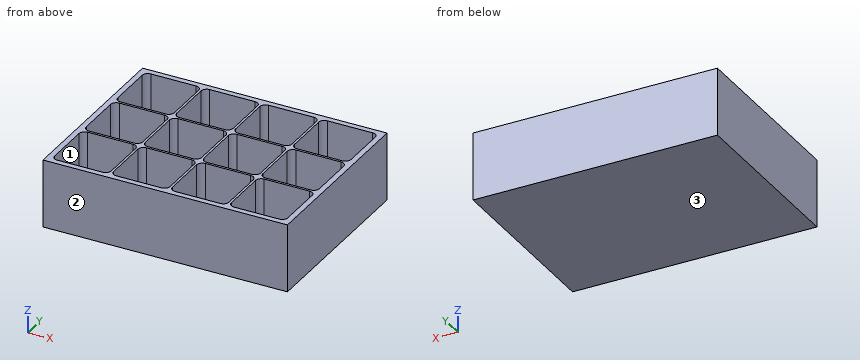
from build123d import *

# Parameters (mm, degrees)
F0_W     = 216
F0_H     = 164
F1_DEPTH = 60
F3_DEPTH = 58


with BuildPart() as f1:
    # F0 (on Top) → F1 (new body)
    with BuildSketch(Plane.XY):
        with Locations((3.771866, 32.061749)):
            Rectangle(F0_W, F0_H)
    extrude(amount=F1_DEPTH)

    # F2 (on face) → F3 (cut)
    with BuildSketch(Plane.XY.offset(60)):
        with BuildLine():
            ThreePointArc((-99.228134, -39.938251), (-97.763668, -43.473785), (-94.228134, -44.938251))
            Line((-94.228134, -44.938251), (-54.228134, -44.938251))
            ThreePointArc((-54.228134, -44.938251), (-50.6926, -43.473785), (-49.228134, -39.938251))
            Line((-49.228134, -39.938251), (-49.228134, 0.061749))
            ThreePointArc((-49.228134, 0.061749), (-50.6926, 3.597283), (-54.228134, 5.061749))
            Line((-54.228134, 5.061749), (-94.228134, 5.061749))
            ThreePointArc((-94.228134, 5.061749), (-97.763668, 3.597283), (-99.228134, 0.061749))
            Line((-99.228134, 0.061749), (-99.228134, -39.938251))
        make_face()
        with BuildLine():
            ThreePointArc((-54.228134, 7.061749), (-50.6926, 8.526215), (-49.228134, 12.061749))
            Line((-49.228134, 12.061749), (-49.228134, 52.061749))
            ThreePointArc((-49.228134, 52.061749), (-50.6926, 55.597283), (-54.228134, 57.061749))
            Line((-54.228134, 57.061749), (-94.228134, 57.061749))
            ThreePointArc((-94.228134, 57.061749), (-97.763668, 55.597283), (-99.228134, 52.061749))
            Line((-99.228134, 52.061749), (-99.228134, 12.061749))
            ThreePointArc((-99.228134, 12.061749), (-97.763668, 8.526215), (-94.228134, 7.061749))
            Line((-94.228134, 7.061749), (-54.228134, 7.061749))
        make_face()
        with BuildLine():
            ThreePointArc((-54.228134, 59.061749), (-50.6926, 60.526215), (-49.228134, 64.061749))
            Line((-49.228134, 64.061749), (-49.228134, 104.061749))
            ThreePointArc((-49.228134, 104.061749), (-50.6926, 107.597283), (-54.228134, 109.061749))
            Line((-54.228134, 109.061749), (-94.228134, 109.061749))
            ThreePointArc((-94.228134, 109.061749), (-97.763668, 107.597283), (-99.228134, 104.061749))
            Line((-99.228134, 104.061749), (-99.228134, 64.061749))
            ThreePointArc((-99.228134, 64.061749), (-97.763668, 60.526215), (-94.228134, 59.061749))
            Line((-94.228134, 59.061749), (-54.228134, 59.061749))
        make_face()
        with BuildLine():
            ThreePointArc((-2.228134, -44.938251), (1.3074, -43.473785), (2.771866, -39.938251))
            Line((2.771866, -39.938251), (2.771866, 0.061749))
            ThreePointArc((2.771866, 0.061749), (1.3074, 3.597283), (-2.228134, 5.061749))
            Line((-2.228134, 5.061749), (-42.228134, 5.061749))
            ThreePointArc((-42.228134, 5.061749), (-45.763668, 3.597283), (-47.228134, 0.061749))
            Line((-47.228134, 0.061749), (-47.228134, -39.938251))
            ThreePointArc((-47.228134, -39.938251), (-45.763668, -43.473785), (-42.228134, -44.938251))
            Line((-42.228134, -44.938251), (-2.228134, -44.938251))
        make_face()
        with BuildLine():
            ThreePointArc((-2.228134, 7.061749), (1.3074, 8.526215), (2.771866, 12.061749))
            Line((2.771866, 12.061749), (2.771866, 52.061749))
            ThreePointArc((2.771866, 52.061749), (1.3074, 55.597283), (-2.228134, 57.061749))
            Line((-2.228134, 57.061749), (-42.228134, 57.061749))
            ThreePointArc((-42.228134, 57.061749), (-45.763668, 55.597283), (-47.228134, 52.061749))
            Line((-47.228134, 52.061749), (-47.228134, 12.061749))
            ThreePointArc((-47.228134, 12.061749), (-45.763668, 8.526215), (-42.228134, 7.061749))
            Line((-42.228134, 7.061749), (-2.228134, 7.061749))
        make_face()
        with BuildLine():
            ThreePointArc((-2.228134, 59.061749), (1.3074, 60.526215), (2.771866, 64.061749))
            Line((2.771866, 64.061749), (2.771866, 104.061749))
            ThreePointArc((2.771866, 104.061749), (1.3074, 107.597283), (-2.228134, 109.061749))
            Line((-2.228134, 109.061749), (-42.228134, 109.061749))
            ThreePointArc((-42.228134, 109.061749), (-45.763668, 107.597283), (-47.228134, 104.061749))
            Line((-47.228134, 104.061749), (-47.228134, 64.061749))
            ThreePointArc((-47.228134, 64.061749), (-45.763668, 60.526215), (-42.228134, 59.061749))
            Line((-42.228134, 59.061749), (-2.228134, 59.061749))
        make_face()
        with BuildLine():
            ThreePointArc((49.771866, -44.938251), (53.3074, -43.473785), (54.771866, -39.938251))
            Line((54.771866, -39.938251), (54.771866, 0.061749))
            ThreePointArc((54.771866, 0.061749), (53.3074, 3.597283), (49.771866, 5.061749))
            Line((49.771866, 5.061749), (9.771866, 5.061749))
            ThreePointArc((9.771866, 5.061749), (6.236332, 3.597283), (4.771866, 0.061749))
            Line((4.771866, 0.061749), (4.771866, -39.938251))
            ThreePointArc((4.771866, -39.938251), (6.236332, -43.473785), (9.771866, -44.938251))
            Line((9.771866, -44.938251), (49.771866, -44.938251))
        make_face()
        with BuildLine():
            ThreePointArc((49.771866, 7.061749), (53.3074, 8.526215), (54.771866, 12.061749))
            Line((54.771866, 12.061749), (54.771866, 52.061749))
            ThreePointArc((54.771866, 52.061749), (53.3074, 55.597283), (49.771866, 57.061749))
            Line((49.771866, 57.061749), (9.771866, 57.061749))
            ThreePointArc((9.771866, 57.061749), (6.236332, 55.597283), (4.771866, 52.061749))
            Line((4.771866, 52.061749), (4.771866, 12.061749))
            ThreePointArc((4.771866, 12.061749), (6.236332, 8.526215), (9.771866, 7.061749))
            Line((9.771866, 7.061749), (49.771866, 7.061749))
        make_face()
        with BuildLine():
            ThreePointArc((49.771866, 59.061749), (53.3074, 60.526215), (54.771866, 64.061749))
            Line((54.771866, 64.061749), (54.771866, 104.061749))
            ThreePointArc((54.771866, 104.061749), (53.3074, 107.597283), (49.771866, 109.061749))
            Line((49.771866, 109.061749), (9.771866, 109.061749))
            ThreePointArc((9.771866, 109.061749), (6.236332, 107.597283), (4.771866, 104.061749))
            Line((4.771866, 104.061749), (4.771866, 64.061749))
            ThreePointArc((4.771866, 64.061749), (6.236332, 60.526215), (9.771866, 59.061749))
            Line((9.771866, 59.061749), (49.771866, 59.061749))
        make_face()
        with BuildLine():
            ThreePointArc((101.771866, -44.938251), (105.3074, -43.473785), (106.771866, -39.938251))
            Line((106.771866, -39.938251), (106.771866, 0.061749))
            ThreePointArc((106.771866, 0.061749), (105.3074, 3.597283), (101.771866, 5.061749))
            Line((101.771866, 5.061749), (61.771866, 5.061749))
            ThreePointArc((61.771866, 5.061749), (58.236332, 3.597283), (56.771866, 0.061749))
            Line((56.771866, 0.061749), (56.771866, -39.938251))
            ThreePointArc((56.771866, -39.938251), (58.236332, -43.473785), (61.771866, -44.938251))
            Line((61.771866, -44.938251), (101.771866, -44.938251))
        make_face()
        with BuildLine():
            ThreePointArc((101.771866, 7.061749), (105.3074, 8.526215), (106.771866, 12.061749))
            Line((106.771866, 12.061749), (106.771866, 52.061749))
            ThreePointArc((106.771866, 52.061749), (105.3074, 55.597283), (101.771866, 57.061749))
            Line((101.771866, 57.061749), (61.771866, 57.061749))
            ThreePointArc((61.771866, 57.061749), (58.236332, 55.597283), (56.771866, 52.061749))
            Line((56.771866, 52.061749), (56.771866, 12.061749))
            ThreePointArc((56.771866, 12.061749), (58.236332, 8.526215), (61.771866, 7.061749))
            Line((61.771866, 7.061749), (101.771866, 7.061749))
        make_face()
        with BuildLine():
            ThreePointArc((101.771866, 59.061749), (105.3074, 60.526215), (106.771866, 64.061749))
            Line((106.771866, 64.061749), (106.771866, 104.061749))
            ThreePointArc((106.771866, 104.061749), (105.3074, 107.597283), (101.771866, 109.061749))
            Line((101.771866, 109.061749), (61.771866, 109.061749))
            ThreePointArc((61.771866, 109.061749), (58.236332, 107.597283), (56.771866, 104.061749))
            Line((56.771866, 104.061749), (56.771866, 64.061749))
            ThreePointArc((56.771866, 64.061749), (58.236332, 60.526215), (61.771866, 59.061749))
            Line((61.771866, 59.061749), (101.771866, 59.061749))
        make_face()
    extrude(amount=-F3_DEPTH, mode=Mode.SUBTRACT)


solid = f1.part
The listing builds one solid part. Answer for the finished solid, in the listing's coordinates (mm). Face numbers are marked on the shaded views. Coordinates: 2 decimals unless noted, no trailing zeros. Loops run counter-clockwise (first coordinate to the right, second up) from the corner with the lowest first, then second, coordinate; pieces in that order, holes last.
1) Find section C-C on z = 7. Give the number of separate pieces and of enclosed holes in the cut face, then the cut area to 3 significant figures.
2) Find the intervals of material crossed by L1, parallel to Y at x = 91, z = 3.5; L2, parallel to X at y = 14.5, z = 24; L3, parallel to Y at x = 102.5, z = 43, in increasing order.
3) Find section A-A on y = 14.5. Write down the section's boundary in (x, z).
4) A flat-ended cylindrical pin translates along its axis: pin 1 Ø5 at (x, y) = (-12.5, 63) entering from +Z. Find the tip coordinate at first contact, or state that the pin passes through.
5) Determine the mould class of the marked faces 1, 2 and 3 for opening direction Y: pulls with the +Y half, pulls with the -Y half, needs draft (parallel to the pull), parting line crosses it, or undercut.
6) Find section B-B on x = -34.5. Write down the section's boundary in (y, z).
Values:
1. separate pieces: 1
1. enclosed holes: 12
1. area: 5,680 mm2
2. L1: y = -49.94 to -44.94, 5.06 to 7.06, 57.06 to 59.06, 109.06 to 114.06
2. L2: x = -104.23 to -99.23, -49.23 to -47.23, 2.77 to 4.77, 54.77 to 56.77, 106.77 to 111.77
2. L3: y = -49.94 to -44.88, 5.01 to 7.12, 57.01 to 59.12, 109.01 to 114.06
3. outline: (-104.23, 0) - (111.77, 0) - (111.77, 60) - (106.77, 60) - (106.77, 2) - (56.77, 2) - (56.77, 60) - (54.77, 60) - (54.77, 2) - (4.77, 2) - (4.77, 60) - (2.77, 60) - (2.77, 2) - (-47.23, 2) - (-47.23, 60) - (-49.23, 60) - (-49.23, 2) - (-99.23, 2) - (-99.23, 60) - (-104.23, 60) - close
4. pin 1: stops at z = 2
5. face 1: undercut
5. face 2: pulls with the -Y half
5. face 3: needs draft
6. outline: (-49.94, 0) - (114.06, 0) - (114.06, 60) - (109.06, 60) - (109.06, 2) - (59.06, 2) - (59.06, 60) - (57.06, 60) - (57.06, 2) - (7.06, 2) - (7.06, 60) - (5.06, 60) - (5.06, 2) - (-44.94, 2) - (-44.94, 60) - (-49.94, 60) - close
